Work out the finished part from the listing and answer in its coordinate system (mm). Face numbers are marked on the shaded views. A direction names the side the tool comes from. Coordinates: 2 decimals unless noted, no trailing zeros. Order: outer loops, then holes, each group sorted by start corner. A loop starts at its lowest first (then second) coordinate and runs counter-clockwise, first axis right, second up. Notation, with made-up numbers: (-26.5, 72.25) -> (-18.5, 72.25) arc R19 cw to (-18.5, 107.25) -> close; hole circle Ø2 at (-7.5, 8). An arc over 180 degrees is marked (long way). Write item = value, one per line. Start each with the question number.
Q1. The part is cut by section B-B, the plane x = -10. Determine the outline of the cut face in (y, z), plus the area to 3 significant figures.
Q2. For a pull along X with two mould halves and no side action, classify the marked faces 4, 5, 6 and 7 as +X half, -X half, draft (parallel to the pull), parting line (faces both ways), or undercut.
Q3. The part is cut by section A-A, the plane z = 44. Count the separate pieces of the cut face and the enclosed holes in it, plus the area to 3 significant figures.
Q4. The part is cut by section C-C, the plane y = -5.75. Determine the outline of the cut face in (x, z), plus the area to 3 significant figures.
Q5. Which of the six approach directions +Z, -Z, +X, -X, +Y, -Y give full straight-line access (tool end or side, diameter ignored) to the marked faces 1, 2 and 3?
Q6. The part is cut by section D-D, the plane x = 0. Determine the outline of the cut face in (y, z).
Q7. Straight lines are drawn through the part: L1, parallel to X at y = 0, z = 44; L2, parallel to Z at x = 14.5, y = -4.75; L3, parallel to Y at x = 5, z = 1 (3 decimals). For each, find the intervals that lie inside material, in ascending order. Write a range as from..to.
Q8. Flat-ended cylindrical pins translate along their axes: pin 1 (6 mm diameter, centred on x = -11, z = 25.5, fed in from -Y); pin 2 (1 mm diameter, centred on y = -1.5, z = 27, fed in from -X); pin 3 (0.6 mm diameter, centred on y = -1.5, z = 22, fed in from +X); pin 4 (3 mm diameter, centred on x = 10.5, z = 44, fed in from +Y). Find the tip coordinate at first contact, or state that the pin passes through.
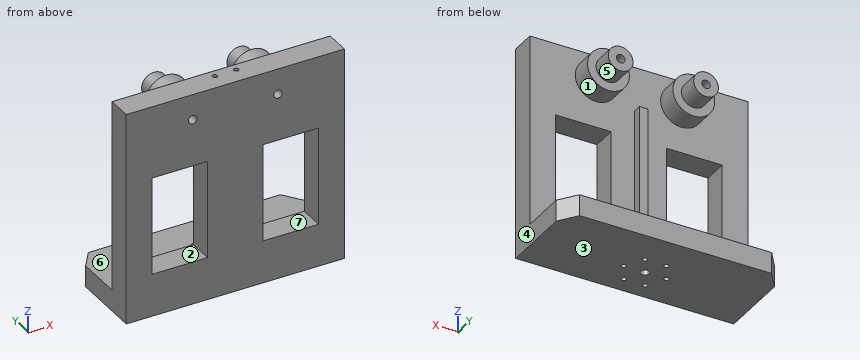
```python
from build123d import *

# Parameters (mm, degrees)
SKETCH1_R               = 1
SKETCH1_R_2             = 0.575
BOSS_EXTRUDE1_DEPTH     = 5
SKETCH2_R               = 0.575
BOSS_EXTRUDE2_DEPTH     = 45
SKETCH4_W               = 2
SKETCH4_H               = 30
BOSS_EXTRUDE3_DEPTH     = 2
SKETCH5_W               = 13
SKETCH5_H               = 23
CUT_EXTRUDE1_DEPTH      = 16
SKETCH6_R               = 2.9
BOSS_EXTRUDE4_DEPTH     = 10
SKETCH7_R               = 1
CUT_EXTRUDE2_DEPTH      = 60.605474742
CUT_EXTRUDE2_DEPTH_BACK = 60.605474742
SKETCH11_R              = 4.9
SKETCH11_R_2            = 2.9
BOSS_EXTRUDE5_DEPTH     = 5
CUT_EXTRUDE4_DEPTH      = 73.577548022
CUT_EXTRUDE4_DEPTH_BACK = 73.577548022


with BuildPart() as part:
    # Sketch1 → Boss-Extrude1 (new body)
    with BuildSketch(Plane.XY):
        Polygon((-22.5, 12.5), (22.5, 12.5), (25.550198027, 8.301762582), (25.550198027, -8.301762582), (22.5, -12.5), (-22.5, -12.5), (-25.550198027, -8.301762582), (-25.550198027, 8.301762582), align=None)
        Circle(SKETCH1_R, mode=Mode.SUBTRACT)
        with Locations((-5, 0)):
            Circle(SKETCH1_R_2, mode=Mode.SUBTRACT)
        with Locations((-2.5, 4.330127019)):
            Circle(SKETCH1_R_2, mode=Mode.SUBTRACT)
        with Locations((2.5, 4.330127019)):
            Circle(SKETCH1_R_2, mode=Mode.SUBTRACT)
        with Locations((5, 0)):
            Circle(SKETCH1_R_2, mode=Mode.SUBTRACT)
        with Locations((2.5, -4.330127019)):
            Circle(SKETCH1_R_2, mode=Mode.SUBTRACT)
        with Locations((-2.5, -4.330127019)):
            Circle(SKETCH1_R_2, mode=Mode.SUBTRACT)
    extrude(amount=BOSS_EXTRUDE1_DEPTH)

    # Sketch2 → Boss-Extrude2 (add)
    with BuildSketch(Plane.XY.offset(5)):
        Polygon((25.550198027, -2.5), (-25.550198027, -2.5), (-25.550198027, -8.301762582), (-22.5, -12.5), (22.5, -12.5), (25.550198027, -8.301762582), align=None)
        with Locations((-2.5, -4.330127019)):
            Circle(SKETCH2_R, mode=Mode.SUBTRACT)
        with Locations((2.5, -4.330127019)):
            Circle(SKETCH2_R, mode=Mode.SUBTRACT)
    extrude(amount=BOSS_EXTRUDE2_DEPTH)

    # Sketch4 → Boss-Extrude3 (add)
    with BuildSketch(Plane(origin=(0, -2.5, 0), x_dir=(1, 0, 0), z_dir=(0, 1, 0))):
        with Locations((0, -24.628925384)):
            Rectangle(SKETCH4_W, SKETCH4_H)
    extrude(amount=BOSS_EXTRUDE3_DEPTH)

    # Sketch5 → Cut-Extrude1 (cut)
    with BuildSketch(Plane(origin=(0, -2.5, 0), x_dir=(1, 0, 0), z_dir=(0, 1, 0))):
        with Locations((13, -21.5)):
            Rectangle(SKETCH5_W, SKETCH5_H)
        with Locations((-13, -21.5)):
            Rectangle(SKETCH5_W, SKETCH5_H)
    extrude(amount=-CUT_EXTRUDE1_DEPTH, mode=Mode.SUBTRACT)

    # Sketch6 → Boss-Extrude4 (add)
    with BuildSketch(Plane(origin=(0, -2.5, 0), x_dir=(1, 0, 0), z_dir=(0, 1, 0))):
        with Locations(Location((10, -44, 0), (0, 0, 270))):
            Circle(SKETCH6_R)
        with Locations(Location((-10, -44, 0), (0, 0, 90))):
            Circle(SKETCH6_R)
    extrude(amount=BOSS_EXTRUDE4_DEPTH)

    # Sketch7 → Cut-Extrude2 (cut, two sides)
    with BuildSketch(Plane(origin=(0, 7.5, 0), x_dir=(1, 0, 0), z_dir=(0, 1, 0))) as cut_extrude2_sk:
        with Locations(Location((10, -44, 0), (0, 0, 270))):
            Circle(SKETCH7_R)
        with Locations(Location((-10, -44, 0), (0, 0, 270))):
            Circle(SKETCH7_R)
    extrude(amount=CUT_EXTRUDE2_DEPTH, mode=Mode.SUBTRACT)
    extrude(cut_extrude2_sk.sketch, amount=-CUT_EXTRUDE2_DEPTH_BACK, mode=Mode.SUBTRACT)

    # Sketch11 → Boss-Extrude5 (add)
    with BuildSketch(Plane(origin=(0, -2.5, 0), x_dir=(1, 0, 0), z_dir=(0, 1, 0))):
        with Locations(Location((-10, -44, 0), (0, 0, 270))):
            Circle(SKETCH11_R)
        with Locations(Location((-10, -44, 0), (0, 0, 90))):
            Circle(SKETCH11_R_2, mode=Mode.SUBTRACT)
        with Locations(Location((10, -44, 0), (0, 0, 270))):
            Circle(SKETCH11_R)
        with Locations(Location((10, -44, 0), (0, 0, 270))):
            Circle(SKETCH11_R_2, mode=Mode.SUBTRACT)
    extrude(amount=BOSS_EXTRUDE5_DEPTH)

    # Sketch13 → Cut-Extrude4 (cut, two sides)
    with BuildSketch(Plane.ZY.offset(25.550198027)) as cut_extrude4_sk:
        Polygon((0, -8.301762582), (-5.234948532, -12.24807669), (12.300258877, -20.537447465), (51.143400136, -17.827460865), (57.147880249, -8.301762582), (50, -8.301762582), align=None)
    extrude(amount=CUT_EXTRUDE4_DEPTH, mode=Mode.SUBTRACT)
    extrude(cut_extrude4_sk.sketch, amount=-CUT_EXTRUDE4_DEPTH_BACK, mode=Mode.SUBTRACT)


solid = part.part
```
Model answer:
q1.outline = (-8.3, 0) -> (12.5, 0) -> (12.5, 5) -> (-2.5, 5) -> (-2.5, 10) -> (-8.3, 10) -> close; (-8.3, 33) -> (-2.5, 33) -> (-2.5, 39.1) -> (2.5, 39.1) -> (2.5, 41.1) -> (7.5, 41.1) -> (7.5, 43) -> (-8.3, 43) -> close; (-8.3, 45) -> (7.5, 45) -> (7.5, 46.9) -> (2.5, 46.9) -> (2.5, 48.9) -> (-2.5, 48.9) -> (-2.5, 50) -> (-8.3, 50) -> close
q1.area = 278 mm2
q2.face_4 = +X half
q2.face_5 = undercut
q2.face_6 = draft
q2.face_7 = undercut
q3.separate_pieces = 3
q3.enclosed_holes = 2
q3.area = 387 mm2
q4.outline = (-25.55, 0) -> (25.55, 0) -> (25.55, 50) -> (-25.55, 50) -> close; hole (-19.5, 10) -> (-6.5, 10) -> (-6.5, 33) -> (-19.5, 33) -> close; hole circle Ø2 at (-10, 44); hole (6.5, 10) -> (19.5, 10) -> (19.5, 33) -> (6.5, 33) -> close; hole circle Ø2 at (10, 44)
q4.area = 1,950 mm2
q5.face_1 = +Y
q5.face_2 = +Y, -Y
q5.face_3 = -Z, +X, -X, +Y, -Y
q6.outline = (-8.3, 0) -> (-1, 0) -> (-1, 5) -> (-2.5, 5) -> (-2.5, 9.63) -> (-0.5, 9.63) -> (-0.5, 39.63) -> (-2.5, 39.63) -> (-2.5, 50) -> (-8.3, 50) -> close; (1, 0) -> (12.5, 0) -> (12.5, 5) -> (1, 5) -> close
q7.L1 = -14.9..-11, -9..-5.1, 5.1..9, 11..14.9
q7.L2 = 0..10, 33..50
q7.L3 = -8.302..-0.575, 0.575..12.5
q8.pin_1 = through
q8.pin_2 = -1
q8.pin_3 = 1
q8.pin_4 = 7.5
